```python
from build123d import *

# Parameters (mm, degrees)
BOSS_EXTRUDE1_DEPTH = 15.1765
SKETCH3_W           = 41
SKETCH3_H           = 20.5
CUT_EXTRUDE1_DEPTH  = 27.178
SKETCH4_R           = 1.905
CUT_EXTRUDE2_DEPTH  = 12.7
SKETCH5_W           = 6.35
SKETCH5_H           = 9.525
CUT_EXTRUDE3_DEPTH  = 10.25


with BuildPart() as part:
    # Sketch2 → Boss-Extrude1 (new, symmetric)
    with BuildSketch(Plane.XY):
        with BuildLine():
            Line((23.765883374, 13.425), (-24.4, 13.425))
            ThreePointArc((-24.4, 13.425), (-28.890128061, 11.565128061), (-30.75, 7.075))
            Line((-30.75, 7.075), (-30.75, -7.075))
            ThreePointArc((-30.75, -7.075), (-28.890128061, -11.565128061), (-24.4, -13.425))
            Line((-24.4, -13.425), (23.765883374, -13.425))
            ThreePointArc((23.765883374, -13.425), (28.256011435, -11.565128061), (30.115883374, -7.075))
            Line((30.115883374, -7.075), (30.115883374, 7.075))
            ThreePointArc((30.115883374, 7.075), (28.256011435, 11.565128061), (23.765883374, 13.425))
        make_face()
    extrude(amount=BOSS_EXTRUDE1_DEPTH, both=True)

    # Sketch3 → Cut-Extrude1 (cut)
    with BuildSketch(Plane.XY.offset(15.1765)):
        Rectangle(SKETCH3_W, SKETCH3_H)
    extrude(amount=-CUT_EXTRUDE1_DEPTH, mode=Mode.SUBTRACT)

    # Sketch4 → Cut-Extrude2 (cut)
    with BuildSketch(Plane.XY.offset(15.1765)):
        with Locations((-24.75, 5)):
            Circle(SKETCH4_R)
        with Locations((-24.75, -5)):
            Circle(SKETCH4_R)
        with Locations((24.75, -5)):
            Circle(SKETCH4_R)
        with Locations((24.75, 5)):
            Circle(SKETCH4_R)
    extrude(amount=-CUT_EXTRUDE2_DEPTH, mode=Mode.SUBTRACT)

    # Sketch5 → Cut-Extrude3 (cut)
    with BuildSketch(Plane.ZY.offset(30.75)):
        with Locations((-7.1755, 0)):
            Rectangle(SKETCH5_W, SKETCH5_H)
    extrude(amount=-CUT_EXTRUDE3_DEPTH, mode=Mode.SUBTRACT)


solid = part.part
```
Here's how the part is built. I have some questions about the finished solid (model axes, mm). A direction names the side the tool comes from. Coordinates: 2 decimals unless noted, no trailing zeros. Loops run counter-clockwise (first coordinate to the right, second up) from the corner with the lowest first, then second, coordinate; pieces in that order, holes last. Notation, with made-up numbers: (-37, 17) - (-25, 17) arc R24 cw to (-25, 27) - close; hole circle Ø3 at (65.25, -15). An arc over 180 degrees is marked (long way). Return JSON: item names as keys, results as strings. Group by question number.
Item 1: If we section it at A-A on z = -11: Write out the boundary of the cut face in (x, y) (3 decimals), and give its area (3 significant figures).
Item 2: If we section it at B-B on z = 8: Write out the boundary of the cut face in (x, y) (3 decimals).
Item 3: I need wall thicknesses on line 1 (Z direction, x = -22.5, y = 3.5); line 2 (X direction, y = 5, z = -3); line 3 (Y direction, x = -22, z = -5) (1 decimal). Which ranges of each line are inside material? Lowest first, please. Write a range as from..to.
Item 4: If we section it at D-D on y = 8.25: Write out the boundary of the cut face in (x, z).
Item 5: We'd pull the mould along X, two halves only. Please class faces 1 (the face through (-8, 12, 15.176)), 2 (the face through (25, -5, 2.477)), 3 (the face through (28.305, 11.515, 0.212)): +X half, -X half, draft (parallel to the pull), parting line (faces both ways), or undercut.
Item 6: On a 3-axis mill with a long thin cutter (end or side, diameter ignored), from which of +Z, -Z, +X, -X, +Y, -Y can I reach the whole of each face in a straight line? I mean faces 4 (the face through (-20.5, 0, 5)), 5 (the face through (-1, -13.425, 0)), 6 (the face through (-26, -4.762, -7)). Say none if no direction works.
Item 7: Will these pins go through, and if not, where does the flat tip stop? P1, Ø1, axis at y = -9, z = 2.5, coming from the +X side; P2, Ø2, axis at y = 10.5, z = -8.5, coming from the +X side.
Calculated:
{
 "1": {"outline": "(-30.75, -7.075) arc R6.35 ccw to (-24.4, -13.425) - (23.766, -13.425) arc R6.35 ccw to (30.116, -7.075) - (30.116, 7.075) arc R6.35 ccw to (23.766, 13.425) - (-24.4, 13.425) arc R6.35 ccw to (-30.75, 7.075) - close; hole (-20.5, -10.25) - (20.5, -10.25) - (20.5, 10.25) - (-20.5, 10.25) - close", "area": "759 mm^2"},
 "2": {"outline": "(-30.75, -7.075) arc R6.35 ccw to (-24.4, -13.425) - (23.766, -13.425) arc R6.35 ccw to (30.116, -7.075) - (30.116, 7.075) arc R6.35 ccw to (23.766, 13.425) - (-24.4, 13.425) arc R6.35 ccw to (-30.75, 7.075) - close; hole circle Ø3.81 at (-24.75, -5); hole circle Ø3.81 at (-24.75, 5); hole (-20.5, -10.25) - (20.5, -10.25) - (20.5, 10.25) - (-20.5, 10.25) - close; hole circle Ø3.81 at (24.75, -5); hole circle Ø3.81 at (24.75, 5)"},
 "3": {"line 1": "z = -15.18..-10.35, -4..15.18", "line 2": "x = -30.75..-20.5, 20.5..30.12", "line 3": "y = -13.4..-4.8, 4.8..13.4"},
 "4": {"outline": "(-30.64, -15.18) - (30.01, -15.18) - (30.01, 15.18) - (20.5, 15.18) - (20.5, -12) - (-20.5, -12) - (-20.5, 15.18) - (-30.64, 15.18) - close"},
 "5": {"face 1": "draft", "face 2": "undercut", "face 3": "+X half"},
 "6": {"face 4": "+Z", "face 5": "+Z, -Z, +X, -X, -Y", "face 6": "-X"},
 "7": {"P1": "stops at x = 29.95", "P2": "stops at x = 29.63"}
}
